Work out the finished part from the listing and answer in its coordinate system (mm). Face numbers are marked on the shaded views. Give positions to 0.01 mm unless a question says otherwise; leave off trailing zeros. Order: outer loops, then holes, each group sorted by start corner. A loop starts at its lowest first (then second) coordinate and runs counter-clockwise, first axis right, second up. Notation, with made-up numbers: (40.5, 85.25) - (95.5, 85.25) arc R27 cw to (95.5, 119.25) - close; hole circle Ø7 at (78.5, 69). An arc over 180 degrees is marked (long way). Put each result on its own line as item: value.
```python
from build123d import *

# Parameters (mm, degrees)
SZKIC1_R                    = 35
DODANIE_WYCI_GNI_CIE1_DEPTH = 6
SZKIC3_R                    = 21.5
WYTNIJ_WYCI_GNI_CIE1_DEPTH  = 6
SZKIC4_R                    = 1.55
WYTNIJ_WYCI_GNI_CIE2_DEPTH  = 6


with BuildPart() as part:
    # Szkic1 → Dodanie-wyciągnięcie1 (new body)
    with BuildSketch(Plane.XY):
        with Locations((41.719839871, 20.384670663)):
            Circle(SZKIC1_R)
    extrude(amount=DODANIE_WYCI_GNI_CIE1_DEPTH)

    # Szkic3 → Wytnij-wyciągnięcie1 (cut)
    with BuildSketch(Plane.XY.offset(6)):
        with Locations((44.619839871, 20.384670663)):
            Circle(SZKIC3_R)
    extrude(amount=-WYTNIJ_WYCI_GNI_CIE1_DEPTH, mode=Mode.SUBTRACT)

    # Szkic4 → Wytnij-wyciągnięcie2 (cut)
    with BuildSketch(Plane.XY.offset(6)):
        with Locations((31.119839871, -2.99801524)):
            Circle(SZKIC4_R)
        with Locations((71.619839871, 20.384670663)):
            Circle(SZKIC4_R)
        with Locations((31.119839871, 43.767356565)):
            Circle(SZKIC4_R)
    extrude(amount=-WYTNIJ_WYCI_GNI_CIE2_DEPTH, mode=Mode.SUBTRACT)


solid = part.part
```
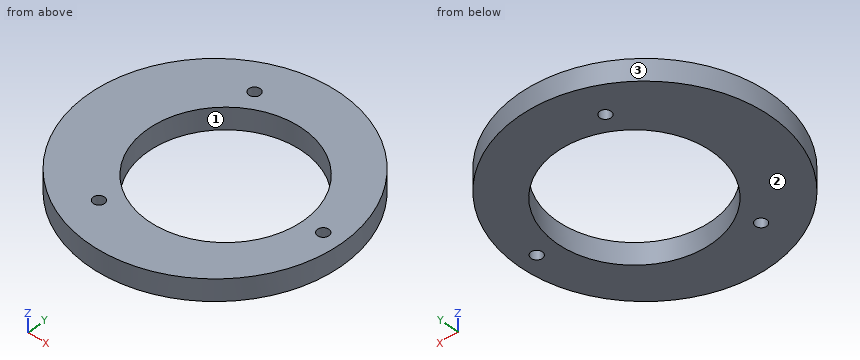
(1) Section B-B, the plane y = 35.5 is taken. Write down the section's boundary in (x, z), then the cut area to 3 significant figures.
Geometry check:
outline: (10.15, 0) - (29.33, 0) - (29.33, 6) - (10.15, 6) - close; (59.91, 0) - (73.29, 0) - (73.29, 6) - (59.91, 6) - close
area: 195 mm²
(2) Section D-D, the plane x = 14 is taken. Write down the section's boundary in (y, z), then the cut area to 3 significant figures.
Geometry check:
outline: (-0.98, 0) - (41.75, 0) - (41.75, 6) - (-0.98, 6) - close
area: 256 mm²
(3) Straight lines are drawn through the part: line 1 (X direction, y = 26.5, z = 1.3); line 2 (X direction, y = 28, z = 0.65); line 3 (Y direction, x = 56, z = 4.7). For each, find the intervals that lie inside material, in ascending order.
Geometry check:
line 1: x = 7.26 to 24.01, 65.23 to 76.18
line 2: x = 7.56 to 24.51, 64.73 to 75.88
line 3: y = -11.57 to 2.14, 38.63 to 52.34
(4) Determine the mould class of the marked faces 1, 2 and 3 for opening direction Y: pulls with the +Y half, pulls with the -Y half, needs draft (parallel to the pull), parting line crosses it, or undercut.
Geometry check:
face 1: undercut
face 2: needs draft
face 3: parting line crosses it
(5) Section A-A, the plane x = 52 is taken. Write down the section's boundary in (y, z).
Geometry check:
outline: (-13.07, 0) - (0.19, 0) - (0.19, 6) - (-13.07, 6) - close; (40.58, 0) - (53.84, 0) - (53.84, 6) - (40.58, 6) - close
(6) Section C-C, the plane z = 2.7 is taken. Write down the section's boundary in (x, y), then the cut area to 3 significant figures.
Geometry check:
outline: circle Ø70 at (41.72, 20.38); hole circle Ø43 at (44.62, 20.38); hole circle Ø3.1 at (31.12, -3); hole circle Ø3.1 at (31.12, 43.77); hole circle Ø3.1 at (71.62, 20.38)
area: 2,370 mm²
(7) Given pin 1 (5 mm diameter, centred on x = 71.62, y = 20.38, fed in from +Z); pin 2 (1 mm diameter, centred on x = 56, z = 5, fed in from +Y), each flat-ended and moving along its own axis, determine where each tip first touches the part or whether it passes through.
Geometry check:
pin 1: stops at z = 6
pin 2: stops at y = 52.56
